Could you check a few things on this model? Use its own coordinates, in mm. Give positions to 0.01 mm unless a question says otherwise; leave off trailing zeros. Order: outer loops, then holes, each group sorted by start corner. A loop starts at its lowest first (then second) coordinate and runs counter-clockwise, first axis right, second up.
(1) Imagine slicing it at B-B, the plane x = 4.3. Write out the boundary of the cut face in (y, z).
(2) Will these pins go through, and if not, where does the flat tip stop? pin 1 (1.8 mm diameter, centred on x = 3.5, y = 72.5, fed in from -Z); pin 2 (2 mm diameter, centred on x = 3, y = 119, fed in from -Z); pin 3 (3 mm diameter, centred on x = 2.5, z = -120.5, fed in from -Y); pin 4 (3 mm diameter, centred on x = 2.5, z = -3.5, fed in from +Y).
(3) If we mould it in two halves opening along Y, with no side actions, what happens to faces 1 (the cylindrical face through (3.042, 119.297, -36.014)), 2 (the flat face through (0, 126, -222))? For each: released by +Y, released by -Y, zero draft, split by the parting line, or undercut.
(4) If I drill on probe 1 along Y at (x, z) = (1.9, -204.5); probe 2 along Z at (x, y) = (4.55, 55); probe 3 along Z at (x, y) = (5.75, 44), over which ranges is the centre line in solid material (lowest first)?
(5) Imagine slicing it at A-A, the plane z = -87.5. Write out the boundary of the cut face in (x, y), then the cut area to 3 significant figures.
(6) Imagine slicing it at C-C, the plane y = 36.5. Write out the boundary of the cut face in (x, z), then the cut area to 3 significant figures.
from build123d import *

# Parameters (mm, degrees)
BOSS_EXTRUDE1_DEPTH = 6
SKETCH2_W           = 6
SKETCH2_H           = 25
CUT_EXTRUDE1_DEPTH  = 6
LPATTERN1_COUNT     = 3
LPATTERN1_PITCH     = 50
FILLET1_R           = 20


with BuildPart() as part:
    # Sketch1 → Boss-Extrude1 (new body)
    with BuildSketch(Plane(origin=(0, 0, 0), x_dir=(0, 0, -1), z_dir=(1, 0, 0))):
        Polygon((450, 125), (450, 150), (0, 150), (0, 0), (450, 0), (450, 27.5), (30, 27.5), (30, 125), align=None)
    extrude(amount=BOSS_EXTRUDE1_DEPTH)

    # Sketch2 → Cut-Extrude1 (cut)
    with BuildSketch(Plane(origin=(6, 0, 0), x_dir=(0, 0, -1), z_dir=(1, 0, 0))):
        with Locations((3, 137.5)):
            Rectangle(SKETCH2_W, SKETCH2_H)
    cut_extrude1 = extrude(amount=-CUT_EXTRUDE1_DEPTH, mode=Mode.SUBTRACT)

    # LPattern1: Cut-Extrude1 ×3
    with Locations(*[(0, -i * LPATTERN1_PITCH, 0) for i in range(1, LPATTERN1_COUNT)]):
        add(cut_extrude1, mode=Mode.SUBTRACT)

    # Fillet1
    fillet1_edges = [part.edges().sort_by_distance(p)[0] for p in [
        (3, 125, -30),
    ]]
    fillet(fillet1_edges, radius=FILLET1_R)


solid = part.part
Answer block:
1. outline: (0, -450) - (27.5, -450) - (27.5, -30) - (105, -30) arc R20 cw to (125, -50) - (125, -450) - (150, -450) - (150, -6) - (125, -6) - (125, 0) - (100, 0) - (100, -6) - (75, -6) - (75, 0) - (50, 0) - (50, -6) - (25, -6) - (25, 0) - (0, 0) - close
2. pin 1: stops at z = -30
2. pin 2: stops at z = -36.77
2. pin 3: stops at y = 0
2. pin 4: stops at y = 125
3. face 1: undercut
3. face 2: zero draft
4. probe 1: y = 0 to 27.5, 125 to 150
4. probe 2: z = -30 to 0
4. probe 3: z = -30 to -6
5. outline: (0, 0) - (6, 0) - (6, 27.5) - (0, 27.5) - close; (0, 125) - (6, 125) - (6, 150) - (0, 150) - close
5. area: 315 mm2
6. outline: (0, -30) - (6, -30) - (6, -6) - (0, -6) - close
6. area: 144 mm2
